Study the drawing (mm; zero at the part's minimum x, y, z) and answer. A direction names the side the tool comes from. Give positions to 0.01 mm unless a question says otherwise; leave off trailing zeros. Write each loop counter-clockwise with the first axis right and the second up, starting at its lowest first coordinate (ties: lowest second). Pieces come first, ordered by that corner, then holes. Notation, with made-up numbers: (40.5, 52) - (89.5, 52) arc R31 cw to (89.5, 84) - close; hole circle Ø4 at (48, 47.25). An arc over 180 degrees is marked (long way). Write each question's results on one line, items separated by ' | '. Start each with the question number.
Q1. For a pull along X with two mould halves and no side action, classify the marked faces 1, 2, 3 and 4 as pulls with the +X half, pulls with the -X half, needs draft (parallel to the pull), parting line crosses it, or undercut.
Q2. Section D-D (y = 19.75) is taken. Determine the outline of the cut face in (x, z).
Q3. Flat-ended cylindrical pins translate along their axes: pin 1 Ø8 at (x, z) = (32, 23.5) entering from +Y; pin 2 Ø10 at (y, z) = (8, 17) entering from +X; pin 3 Ø2 at (x, y) = (32, 24.5) entering from -Z. Find the tip coordinate at first contact, or state that the pin passes through.
Q4. Section B-B (y = 15) is taken. Determine the outline of the cut face in (x, z), plus the area to 3 significant figures.
Q5. Find the intervals of material crossed by probe 1 along Y at (x, z) = (2.2, 15); probe 2 along X at (y, z) = (8.75, 5.5); probe 3 along Z at (x, y) = (29, 12.5), in increasing order.
Q6. For the marked faces 5 and 6, determine the directions among +Z, -Z, +X, -X, +Y, -Y from which every point of the face is accessible in a straight line to the end or side of a thin tool.
Q7. Section A-A (x = 15) is taken. Determine the outline of the cut face in (y, z).
Q8. Section C-C (z = 15) is taken. Determine the outline of the cut face in (x, y), plus the area to 3 significant figures.
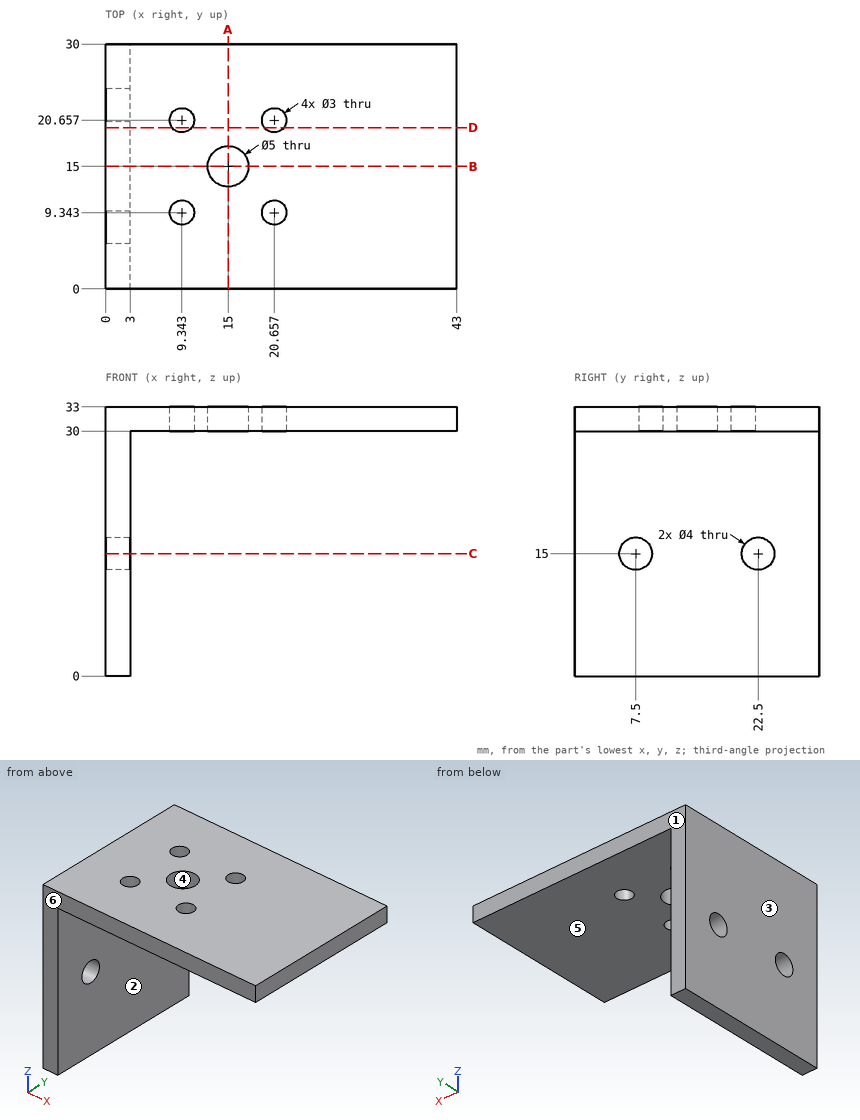
Answers below:
1) face 1: needs draft | face 2: pulls with the +X half | face 3: pulls with the -X half | face 4: undercut
2) outline: (0, 0) - (3, 0) - (3, 30) - (8.15, 30) - (8.15, 33) - (0, 33) - close; (10.54, 30) - (19.46, 30) - (19.46, 33) - (10.54, 33) - close; (21.85, 30) - (43, 30) - (43, 33) - (21.85, 33) - close
3) pin 1: passes through | pin 2: stops at x = 3 | pin 3: stops at z = 30
4) outline: (0, 0) - (3, 0) - (3, 30) - (12.5, 30) - (12.5, 33) - (0, 33) - close; (17.5, 30) - (43, 30) - (43, 33) - (17.5, 33) - close | area: 204 mm2
5) probe 1: y = 0 to 5.5, 9.5 to 20.5, 24.5 to 30 | probe 2: x = 0 to 3 | probe 3: z = 30 to 33
6) face 5: -Z, +X, +Y, -Y | face 6: +Z, -Z, +X, -X, -Y
7) outline: (0, 30) - (12.5, 30) - (12.5, 33) - (0, 33) - close; (17.5, 30) - (30, 30) - (30, 33) - (17.5, 33) - close
8) outline: (0, 0) - (3, 0) - (3, 5.5) - (0, 5.5) - close; (0, 9.5) - (3, 9.5) - (3, 20.5) - (0, 20.5) - close; (0, 24.5) - (3, 24.5) - (3, 30) - (0, 30) - close | area: 66.0 mm2
